Autodesk Inventor part; units mm, degrees
ref_plane "YZ Plane" through (0, 0, 0) normal (1, 0, 0) x (0, 1, 0)
ref_plane "XZ Plane" through (0, 0, 0) normal (0, 1, 0) x (-1, 0, 0)
ref_plane "XY Plane" through (0, 0, 0) normal (0, 0, 1) x (1, 0, 0)
sketch "Sketch1" plane through (0, 0, 0) normal (0, 0, 1) x (1, 0, 0)
  line L0 (0, 7.3323) -> (6.35, 3.6662)
  line L1 (6.35, 3.6662) -> (6.35, -3.6662)
  line L2 (6.35, -3.6662) -> (0, -7.3323)
  line L3 (0, -7.3323) -> (-6.35, -3.6662)
  line L4 (-6.35, -3.6662) -> (-6.35, 3.6662)
  line L5 (-6.35, 3.6662) -> (0, 7.3323)
  circle A0 centre (0, 23.8125) radius 2.159
  circle A1 centre (0, 0) radius 19.05
  circle A2 centre (0, 23.8125) radius 4.7625
  circle A3 centre (-20.6222, 11.9063) radius 4.7625
  circle A4 centre (-20.6222, 11.9063) radius 2.159
  circle A5 centre (-20.6222, -11.9062) radius 4.7625
  circle A6 centre (-20.6222, -11.9062) radius 2.159
  circle A7 centre (0, -23.8125) radius 4.7625
  circle A8 centre (0, -23.8125) radius 2.159
  circle A9 centre (20.6222, -11.9063) radius 4.7625
  circle A10 centre (20.6222, -11.9063) radius 2.159
  circle A11 centre (20.6222, 11.9062) radius 4.7625
  circle A12 centre (20.6222, 11.9062) radius 2.159
  arc A13 (-7.466, 17.526) -> (-4.6663, 22.86) centre (-9.3326, 21.9075) ccw
  arc A14 (4.6663, 22.86) -> (7.466, 17.526) centre (9.3326, 21.9075) ccw
  arc A15 (-18.911, 2.2972) -> (-22.1305, 7.3889) centre (-23.6387, 2.8715) ccw
  arc A16 (-17.4642, 15.4711) -> (-11.4449, 15.2288) centre (-14.3062, 19.036) ccw
  arc A17 (-11.4449, -15.2288) -> (-17.4642, -15.4711) centre (-14.3062, -19.036) ccw
  arc A18 (-22.1305, -7.3889) -> (-18.911, -2.2972) centre (-23.6387, -2.8715) ccw
  arc A19 (7.466, -17.526) -> (4.6663, -22.86) centre (9.3326, -21.9075) ccw
  arc A20 (-4.6663, -22.86) -> (-7.466, -17.526) centre (-9.3326, -21.9075) ccw
  arc A21 (18.911, -2.2972) -> (22.1305, -7.3889) centre (23.6387, -2.8715) ccw
  arc A22 (17.4642, -15.4711) -> (11.4449, -15.2288) centre (14.3062, -19.036) ccw
  arc A23 (11.4449, 15.2288) -> (17.4642, 15.4711) centre (14.3062, 19.036) ccw
  arc A24 (22.1305, 7.3889) -> (18.911, 2.2972) centre (23.6387, 2.8715) ccw
  point P0 (0, 19.05)
  point P1 (-3.6714, 18.6929)
  point P2 (-16.4978, 9.525)
  point P3 (-18.0242, 6.1669)
  point P4 (-16.4978, -9.525)
  point P5 (-14.3528, -12.526)
  point P6 (0, -19.05)
  point P7 (3.6714, -18.6929)
  point P8 (16.4978, -9.525)
  point P9 (18.0242, -6.1669)
  point P10 (16.4978, 9.525)
  point P11 (14.3528, 12.526)
  point P12 (22.1305, 7.3889)
  point P13 (11.4449, -15.2288)
  point P14 (17.4642, -15.4711)
  point P15 (22.1305, -7.3889)
  point P16 (-7.466, -17.526)
  point P17 (-4.6663, -22.86)
  point P18 (4.6663, -22.86)
  point P19 (-18.911, -2.2972)
  point P20 (-22.1305, -7.3889)
  point P21 (-17.4642, -15.4711)
  point P22 (-11.4449, -15.2288)
  point P23 (-11.4449, 15.2288)
  point P24 (-22.1305, 7.3889)
  dimension "d0" = 12.7
  dimension "d1" = 4.318
  dimension "d2" = 38.1
  dimension "d3" = 9.525
  dimension "d6" = 360
  dimension "d11" = 23.8125
  dimension "d14" = 360
extrude "Extrusion1" add sketch "Sketch1" along normal blind 6.35
properties part number "HubPlate" material "Aluminum 6061"
The listing builds one solid part. Answer for the finished solid, in the listing's coordinates (mm). A direction names the side the tool comes from. Coordinates: 2 decimals unless noted, no trailing zeros. Write each loop counter-clockwise with the first axis right and the second up, starting at its lowest first coordinate (ties: lowest second). Pieces come first, ordered by that corner, then holes. Notation, with made-up numbers: (31, -6) - (73, -6) arc R12 cw to (73, 9) - close; hole circle Ø8 at (7, 5.5). An arc over 180 degrees is marked (long way). Return JSON: item names as keys, results as strings. Group by question number.
Q1. The part is cut by section C-C on y = -19. Write down the section's boundary in (x, z), and give its area (3 significant figures).
Q2. The part is cut by section B-B on y = -25. Write down the section's boundary in (x, z).
Q3. Which of the six approach directions +Z, -Z, +X, -X, +Y, -Y give full straight-line access (tool end or side, diameter ignored) to faces 5 (the flat face through (6.35, 0, 3)), 6 (the cylindrical face through (-9.553, 16.482, 3.131)), 7 (the cylindrical face through (19.05, 0.03, 3.13))?
Q4. Find the intervals of material crossed by line 1 along X through (y, z) = (0.5, 0.75); line 2 along X through (y, z) = (15.5, 3.5); line 3 along X through (y, z) = (15, 1.5), in increasing order. Write a range as [from, to].
Q5. The part is cut by section A-A on x = -21.5. Write down the section's boundary in (y, z).
Q6. For a pull along X with two mould halves and no side action, classify faces 1 (the cylindrical face through (5.14, 19.65, 3.13)), 2 (the cylindrical face through (19.03, 10.45, 3.13)), 3 (the cylindrical face through (-19.05, -0.03, 3.13)), 4 (the flat face through (-6.35, 0, 3)) as +X half, -X half, draft (parallel to the pull), parting line (faces both ways), or undercut.
Q7. The part is cut by section D-D on x = -14. Write down the section's boundary in (y, z).
Q8. Flat-ended cylindrical pins translate along their axes: pin 1 Ø3 at (x, z) = (-7.5, 3) entering from +Y; pin 2 Ø5.5 at (x, y) = (20.62, 11.91) entering from -Z; pin 3 Ø4 at (x, y) = (20.62, -11.91) entering from -Z; pin 4 Ø3 at (y, z) = (-0.5, 4.5) entering from -X. Find the tip coordinate at first contact, or state that the pin passes through.
Evaluation:
{
 "1": {"outline": "(-5.56, 0) - (5.56, 0) - (5.56, 6.35) - (-5.56, 6.35) - close", "area": "70.6 mm2"},
 "2": {"outline": "(-4.61, 0) - (-1.8, 0) - (-1.8, 6.35) - (-4.61, 6.35) - close; (1.8, 0) - (4.61, 0) - (4.61, 6.35) - (1.8, 6.35) - close"},
 "3": {"face 5": "+Z, -Z", "face 6": "+Z, -Z, +Y", "face 7": "+Z, -Z, +X"},
 "4": {"line 1": "x = [-19.04, -6.35], [6.35, 19.04]", "line 2": "x = [-23.75, -17.5], [-11.07, 11.07], [17.5, 23.75]", "line 3": "x = [-24.24, -16.83], [-11.78, 11.78], [16.83, 24.24]"},
 "5": {"outline": "(-16.59, 0) - (-13.88, 0) - (-13.88, 6.35) - (-16.59, 6.35) - close; (-9.93, 0) - (-7.13, 0) - (-7.13, 6.35) - (-9.93, 6.35) - close; (7.13, 0) - (9.93, 0) - (9.93, 6.35) - (7.13, 6.35) - close; (13.88, 0) - (16.59, 0) - (16.59, 6.35) - (13.88, 6.35) - close"},
 "6": {"face 1": "+X half", "face 2": "undercut", "face 3": "-X half", "face 4": "undercut"},
 "7": {"outline": "(-14.28, 0) - (14.28, 0) - (14.28, 6.35) - (-14.28, 6.35) - close"},
 "8": {"pin 1": "stops at y = 18.51", "pin 2": "stops at z = 0", "pin 3": "passes through", "pin 4": "stops at x = -19.05"}
}
